Check sheet for the modelled part. Datum: model origin and axes. Units: mm. A direction names the side the tool comes from. Round coordinates to 2 decimals unless told otherwise and drop trailing zeros. Loops run counter-clockwise (first coordinate to the right, second up) from the corner with the lowest first, then second, coordinate; pieces in that order, holes last. Notation, with made-up numbers: (27.25, 30) - (66.25, 30) arc R25 cw to (66.25, 46) - close; hole circle Ø10 at (83.25, 64). An arc over 180 degrees is marked (long way). Put each result on its own line as item: value. Start each with the question number.
Item 1: Draft check along Y on faces 1 (the flat face through (3.3, 1, -0.1)), 2 (the cylindrical face through (8.5, -56, -0.1)), 3 (the cylindrical face through (8.51, -52.53, -0.33)). Enter one of: pulls with the +Y half, pulls with the -Y half, needs draft (parallel to the pull), parting line crosses it, or undercut.
Item 2: Material ranges on line 1 along Y through (x, z) = (8.5, 0); line 2 along X through (y, z) = (0.75, 0); line 3 along Z through (x, y) = (8.3, -50), recorded low to high.
Item 3: Section check B-B, the plane y = -48. Record the cut outline in (x, z).
Item 4: Section check D-D, the plane x = 7.25. Record the cut outline in (y, z).
Item 5: Gauge pin test, flat ends, axial feed: pin 1 Ø3 at (x, z) = (1.5, 1) entering from -Y; pin 2 Ø5.5 at (x, z) = (0, 0) entering from +Y; pin 3 Ø4 at (y, z) = (-45.5, -1.5) entering from -X. Record the tip position at first contact, or that the pin passes through.
Item 6: Tool access check on faces 4 (the flat face through (8.2, -18.7, -6)), 5 (the flat face through (8, -28, 0)). Record the directions out of +Z, -Z, +X, -X, +Y, -Y that give a thin tool (end or side, any length) a straight path to the whole face; none if there is none.
Item 7: Section check C-C, the plane x = 2. Record the cut outline in (y, z).
Item 8: Section check A-A, the plane z = 0. Record the cut outline in (x, y).
from build123d import *

# Parameters (mm, degrees)
SKETCH1_R           = 3.05
BOSS_EXTRUDE1_DEPTH = 1
BOSS_EXTRUDE2_START = 9
SKETCH3_R           = 2.55
BOSS_EXTRUDE2_DEPTH = 1


with BuildPart() as part:
    # Sketch1 → Boss-Extrude1 (new body)
    with BuildSketch(Plane(origin=(0, 0, 0), x_dir=(1, 0, 0), z_dir=(0, 1, 0))):
        with BuildLine():
            Line((0, 6), (9, 6))
            Line((9, 6), (9, -6))
            Line((9, -6), (0, -6))
            ThreePointArc((0, -6), (-6, 0), (0, 6))
        make_face()
        with Locations(Location((0, 0, 0), (0, 0, 270))):
            Circle(SKETCH1_R, mode=Mode.SUBTRACT)
    extrude(amount=BOSS_EXTRUDE1_DEPTH)

    # Sketch3 → Boss-Extrude2 (add)
    with BuildSketch(Plane(origin=(0, 0, 0), x_dir=(0, 0, -1), z_dir=(1, 0, 0)).offset(BOSS_EXTRUDE2_START)):
        with BuildLine():
            Line((-6, 0), (6, 0))
            Line((6, 0), (6, -50))
            ThreePointArc((6, -50), (0, -56), (-6, -50))
            Line((-6, -50), (-6, 0))
        make_face()
        with Locations(Location((0, -50, 0), (0, 0, 180))):
            Circle(SKETCH3_R, mode=Mode.SUBTRACT)
    extrude(amount=-BOSS_EXTRUDE2_DEPTH)


solid = part.part
Check result:
1. face 1: pulls with the +Y half
1. face 2: pulls with the -Y half
1. face 3: undercut
2. line 1: -56 to -52.55, -47.45 to 1
2. line 2: -6 to -3.05, 3.05 to 9
2. line 3: -6 to -2.55, 2.55 to 6
3. outline: (8, -6) - (9, -6) - (9, -1.58) - (8, -1.58) - close; (8, 1.58) - (9, 1.58) - (9, 6) - (8, 6) - close
4. outline: (0, -6) - (1, -6) - (1, 6) - (0, 6) - close
5. pin 1: y = 0
5. pin 2: through
5. pin 3: x = 8
6. face 4: -Z, +X, -X, +Y, -Y
6. face 5: +Z, -Z, -X, -Y
7. outline: (0, -6) - (1, -6) - (1, -2.3) - (0, -2.3) - close; (0, 2.3) - (1, 2.3) - (1, 6) - (0, 6) - close
8. outline: (-6, 0) - (-3.05, 0) - (-3.05, 1) - (-6, 1) - close; (3.05, 0) - (8, 0) - (8, -47.45) - (9, -47.45) - (9, 1) - (3.05, 1) - close; (8, -56) - (9, -56) - (9, -52.55) - (8, -52.55) - close
